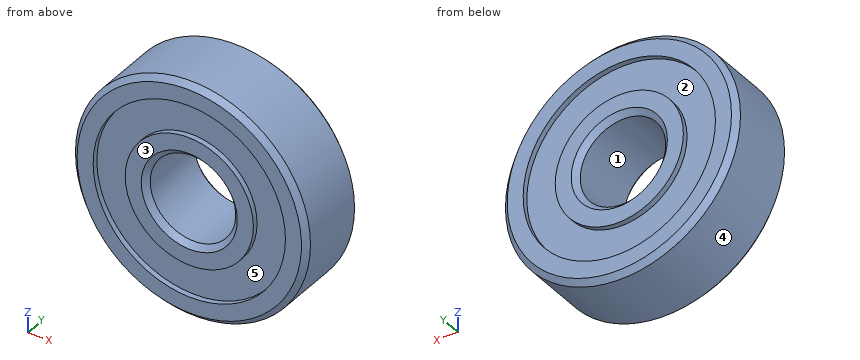
Autodesk Inventor part; units mm, degrees
ref_plane "Work Plane1" through (0, 6.5, 0) normal (0, 1, 0) x (1, 0, 0)
ref_plane "YZ Plane" through (0, 0, 0) normal (1, 0, 0) x (0, 1, 0)
ref_plane "XZ Plane" through (0, 0, 0) normal (0, 1, 0) x (-1, 0, 0)
sketch "Sketch1" plane through (0, 0, 0) normal (0, 1, 0) x (-1, 0, 0)
  circle A0 centre (0, 0) radius 11
  circle A1 centre (0, 0) radius 4
  circle A2 centre (0, 0) radius 6
  circle A3 centre (0, 0) radius 9
  dimension "d0" = 22
  dimension "d1" = 8
  dimension "d2" = 2
  dimension "d3" = 2
extrude "Extrusion1" add sketch "Sketch1" along normal blind 7
ref_plane "Work Plane1" through (0, 6.5, 0) normal (0, 1, 0) x (1, 0, 0)
sketch "Sketch2" plane through (0, 6.5, 0) normal (0, 1, 0) x (1, 0, 0)
  circle A0 centre (0, 0) radius 6
  circle A1 centre (0, 0) radius 9
  circle A2 centre (0, 0) radius 6
  circle A3 centre (0, 0) radius 9
extrude "Extrusion2" add sketch "Sketch2" against normal blind 6
chamfer "Chamfer1" distance 0.5 angle 45 4 edges at (11, 7, 0) (11, 0, 0) (4, 7, 0) (4, 0, 0)
properties part number "Cojinete_608zz"
The listing builds one solid part. Answer for the finished solid, in the listing's coordinates (mm). Face numbers are marked on the shaded views. A direction names the side the tool comes from. Coordinates: 2 decimals unless noted, no trailing zeros. Write each loop counter-clockwise with the first axis right and the second up, starting at its lowest first coordinate (ties: lowest second). Pieces come first, ordered by that corner, then holes. Notation, with made-up numbers: (84.5, 6.25) - (124.5, 6.25) arc R17 cw to (124.5, 21.25) - close; hole circle Ø9 at (25, 1). An arc over 180 degrees is marked (long way). Answer as CSV lines item,"result".
1. Given P1, Ø4, axis at x = -5, y = 4.5, coming from the -Z side; P2, Ø1, axis at y = 2.5, z = 3.5, coming from the -X side; P3, Ø1, axis at y = 2.5, z = -4, coming from the -X side, each flat-ended and moving along its own axis, determine where each tip first touches the part or whether it passes through.
Computed values:
P1,"stops at z = -10.58"
P2,"stops at x = -10.58"
P3,"stops at x = -10.43"
2. Straight lines are drawn through the part: line 1 (Z direction, x = 0, y = 6.95); line 2 (Z direction, x = 0, y = 6.9); line 3 (Y direction, x = 6.25, z = 2.25). For each, find the intervals that lie inside material, in ascending order. Write a range as [from, to].
Computed values:
line 1,"z = [-10.55, -9], [-6, -4.45], [4.45, 6], [9, 10.55]"
line 2,"z = [-10.6, -9], [-6, -4.4], [4.4, 6], [9, 10.6]"
line 3,"y = [0.5, 6.5]"
3. A tool of negligible diameter and unlimited length cuts with its end or side. For the marked faces 1 and 2, from which of +Z, -Z, +X, -X, +Y, -Y can it reach the whole face along a straight path? Write none if from no direction.
Computed values:
face 1,"+Y, -Y"
face 2,"+Y"
4. Determine the mould class of the marked faces 3, 4 and 5 for opening direction X: +X half, -X half, draft (parallel to the pull), parting line (faces both ways), or undercut.
Computed values:
face 3,"draft"
face 4,"parting line"
face 5,"undercut"
5. Find section C-C (y = 5). Give the vertices of the cut face in (x, z).
Computed values:
outline,"circle Ø22 at (0, 0); hole circle Ø8 at (0, 0)"
